Could you check a few things on this model? Use its own coordinates, in mm. Face numbers are marked on the shaded views. A direction names the side the tool comes from. Round coordinates to 2 decimals unless told otherwise and drop trailing zeros. Loops run counter-clockwise (first coordinate to the right, second up) from the corner with the lowest first, then second, coordinate; pieces in that order, holes last. Notation, with made-up numbers: (-30.5, 26) -> (-2.5, 26) arc R23 cw to (-2.5, 49) -> close; hole circle Ø4 at (-33.5, -15.75). An arc over 180 degrees is marked (long way). Write each question's results on one line, items separated by ' | '. Start each with the question number.
1) We'd pull the mould along X, two halves only. Please class the marked faces 3, 4, 5 and 6: pulls with the +X half, pulls with the -X half, needs draft (parallel to the pull), parting line crosses it, or undercut.
2) Which directions (+Z, -Z, +X, -X, +Y, -Y) give clear straight access to the entire face, cutting with the end or side of a thin tool? Please do the marked faces 1 and 2.
3) For P1, Ø1.2, axis at x = 0, y = 0, coming from the -Z side; P2, Ø1, axis at x = 0, y = 0, coming from the +Z side, each with a flat end and sliding along its axis, tell me the tip position at first contact or that it passes through.
4) Imagine slicing it at B-B, the plane x = 1. List the corners of the cut face in (y, z) for me.
5) Imagine slicing it at A-A, the plane z = 5.5. List the corners of the cut face in (x, y) for me, plus the area to 3 significant figures.
6) Imagine slicing it at C-C, the plane z = 8. List the corners of the cut face in (x, y) for me, plus the area to 3 significant figures.
7) If I drill on probe 1 along Y at (x, z) = (1.2, 8); probe 2 along Z at (x, y) = (1, 0); probe 3 along X at (y, z) = (-0.3, 7), over which ranges is the centre line in solid material (lowest first)?
8) Imagine slicing it at D-D, the plane z = 1.25. List the corners of the cut face in (x, y) for me.
Autodesk Inventor part; units mm, degrees
ref_plane "YZ Plane" through (0, 0, 0) normal (1, 0, 0) x (0, 1, 0)
ref_plane "XZ Plane" through (0, 0, 0) normal (0, 1, 0) x (-1, 0, 0)
ref_plane "XY Plane" through (0, 0, 0) normal (0, 0, 1) x (1, 0, 0)
sketch "Skizze1" plane through (0, 0, 0) normal (0, 0, 1) x (1, 0, 0)
  line L0 (-1.5, -1.5) -> (1.5, -1.5)
  line L1 (1.5, -1.5) -> (1.5, 1.5)
  line L2 (1.5, 1.5) -> (-1.5, 1.5)
  line L3 (-1.5, 1.5) -> (-1.5, -1.5)
  line L4 (-1.5, -1.5) -> (1.5, 1.5) construction
  line L5 (1.5, -1.5) -> (-1.5, 1.5) construction
  point P0 (0, 0)
  dimension "d0" = 3
  dimension "d1" = 3
extrude "Extrusion1" add sketch "Skizze1" along normal blind 9
sketch "Skizze2" plane through (0, 0, 9) normal (0, 0, 1) x (1, 0, 0)
  line L0 (0, 0) -> (0, 3.7062) construction
  line L1 (1.5, 1.5) -> (-1.5, 1.5)
  line L2 (-0.6, -1.5) -> (0.6, -1.5)
  line L3 (0.6, -1.5) -> (0.6, 1.5)
  line L4 (0.6, 1.5) -> (-0.6, 1.5)
  line L5 (-0.6, 1.5) -> (-0.6, -1.5)
  line L6 (-1.5, -1.5) -> (1.5, -1.5)
  dimension "d4" = 1.2
extrude "Extrusion2" cut sketch "Skizze2" against normal blind 4
sketch "Skizze3" plane through (1.5, -1.5, 0) normal (1, 0, 0) x (0, 0, -1)
  line L0 (-9, 0) -> (-9, 3)
  line L1 (0, 0) -> (0, 3)
  point P0 (0, 1.5)
  point P1 (-8, 1.5)
  point P2 (-9, 1.5)
  dimension "d14" = 8
hole "Bohrung1" at (1.5, 0, 8) direction (-1, 0, 0) diameter 1 depth 0.9
mirror "Spiegeln1" about plane through (0, 0, 0) normal (1, 0, 0) of "Bohrung1"
sketch "Skizze4" plane through (0, 0, 0) normal (0, 0, -1) x (-1, 0, 0)
  line L0 (-1.5, -1.5) -> (-1.5, 1.5)
  line L1 (1.5, -1.5) -> (-1.5, -1.5)
  point P0 (0, 0)
  point P1 (0, 0)
  point P2 (-1.5, 0)
  point P3 (0, -1.5)
hole "Bohrung2" at (0, 0, 0) direction (0, 0, 1) diameter 1.5 depth 2.5 tip angle 118
chamfer "Fasen1" distance 0.5 angle 45 4 edges at (1.05, -1.5, 9) (1.05, 1.5, 9) (-1.05, 1.5, 9) (-1.05, -1.5, 9)
properties part number "kopf"
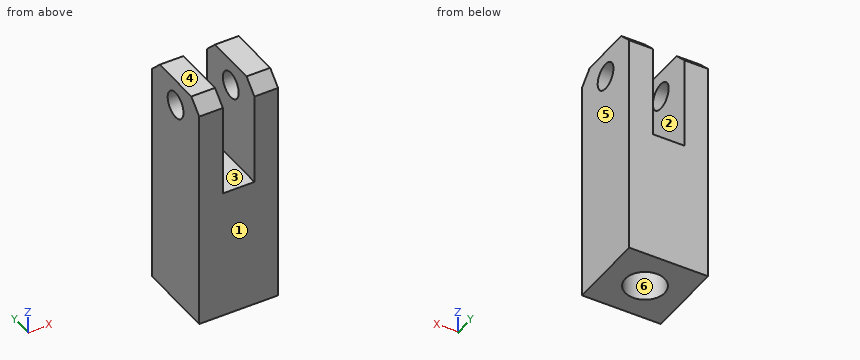
Checked values:
1) face 3: undercut | face 4: needs draft | face 5: pulls with the +X half | face 6: undercut
2) face 1: +Z, -Z, +X, -X, -Y | face 2: +Z, +Y, -Y
3) P1: z = 2.59 | P2: z = 5
4) outline: (-1.5, 0) -> (1.5, 0) -> (1.5, 8.5) -> (1, 9) -> (-1, 9) -> (-1.5, 8.5) -> close; hole circle Ø1 at (0, 8)
5) outline: (-1.5, -1.5) -> (-0.6, -1.5) -> (-0.6, 1.5) -> (-1.5, 1.5) -> close; (0.6, -1.5) -> (1.5, -1.5) -> (1.5, 1.5) -> (0.6, 1.5) -> close | area: 5.40 mm^2
6) outline: (-1.5, -1.5) -> (-0.6, -1.5) -> (-0.6, -0.5) -> (-1.5, -0.5) -> close; (-1.5, 0.5) -> (-0.6, 0.5) -> (-0.6, 1.5) -> (-1.5, 1.5) -> close; (0.6, -1.5) -> (1.5, -1.5) -> (1.5, -0.5) -> (0.6, -0.5) -> close; (0.6, 0.5) -> (1.5, 0.5) -> (1.5, 1.5) -> (0.6, 1.5) -> close | area: 3.60 mm^2
7) probe 1: -1.5 to -0.5, 0.5 to 1.5 | probe 2: 0 to 7.5, 8.5 to 9 | probe 3: -1.5 to -0.6, 0.6 to 1.5
8) outline: (-1.5, -1.5) -> (1.5, -1.5) -> (1.5, 1.5) -> (-1.5, 1.5) -> close; hole circle Ø1.5 at (0, 0)
